Input: part model. Units: mm. Frame: model coordinates. Round coordinates to 2 decimals unless told otherwise and drop trailing zeros. Loops run counter-clockwise (first coordinate to the right, second up) from the corner with the lowest first, then second, coordinate; pieces in that order, holes last. Notation, with made-up numbers: (79, 36.25) -> (97, 36.25) arc R14 ccw to (97, 42.25) -> close; hole circle Ø4 at (50.25, -35.5). An arc over 180 degrees is marked (long way). Answer as a JSON object with one key per item and string values. Group by question number.
Item 1: Section query A-A on z = -255. Return loops of the section in (x, y), and give its area (3 significant figures).
Item 2: Pin query (flat end, axial travel): pin 1 (5.5 mm diameter, centred on y = 12.7, z = 12.7, fed in from +X); pin 2 (4.5 mm diameter, centred on x = 25.4, z = -285.75, fed in from +Y). Return the tip coordinate at first contact, or that it passes through.
Item 3: Material intervals for line 1 (X direction, y = 24.55, z = 31.75); line 2 (Y direction, x = 16, z = -77); line 3 (Y direction, x = 0.85, z = 139.7), sorted ascending. Write a range as [from, to].
Item 4: Section query B-B on y = 19. Return loops of the section in (x, z).
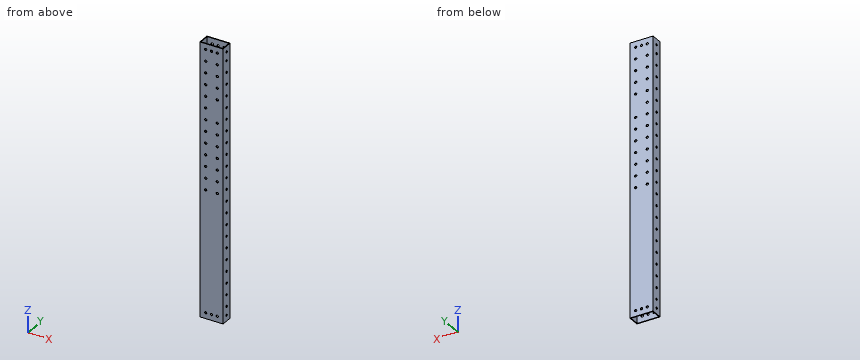
from build123d import *

# Parameters (mm, degrees)
SKETCH1_W           = 50.8
SKETCH1_H           = 25.4
BOSS_EXTRUDE1_DEPTH = 298.45
SHELL1_T            = -1.5875
SKETCH2_R           = 2.4892
CUT_EXTRUDE1_DEPTH  = 304.806192333
SKETCH3_R           = 2.4892
CUT_EXTRUDE2_DEPTH  = 304.806192333
SKETCH4_R           = 2.4892
CUT_EXTRUDE3_DEPTH  = 304.806192333
LPATTERN1_COUNT     = 22
LPATTERN1_PITCH     = 25.4
SKETCH5_R           = 2.4892
CUT_EXTRUDE4_DEPTH  = 304.806192333


with BuildPart() as part:
    # Sketch1 → Boss-Extrude1 (new, symmetric)
    with BuildSketch(Plane.XY):
        with Locations((25.4, 12.7)):
            Rectangle(SKETCH1_W, SKETCH1_H)
    extrude(amount=BOSS_EXTRUDE1_DEPTH, both=True)

    # Shell1
    shell1_openings = [part.faces().sort_by_distance(p)[0] for p in [
        (25.4, 12.7, 298.45),
        (25.4, 12.7, -298.45),
    ]]
    offset(amount=SHELL1_T, openings=shell1_openings, kind=Kind.INTERSECTION)

    # Sketch2 → Cut-Extrude1 (cut, through all)
    with BuildSketch(Plane(origin=(0, 25.4, 0), x_dir=(1, 0, 0), z_dir=(0, 1, 0))):
        with Locations(Location((38.1, -285.75, 0), (0, 0, 270))):
            Circle(SKETCH2_R)
        with Locations(Location((25.4, -285.75, 0), (0, 0, 270))):
            Circle(SKETCH2_R)
        with Locations(Location((12.7, -285.75, 0), (0, 0, 270))):
            Circle(SKETCH2_R)
    cut_extrude1 = extrude(amount=-CUT_EXTRUDE1_DEPTH, mode=Mode.SUBTRACT)

    # Sketch3 → Cut-Extrude2 (cut, through all)
    with BuildSketch(Plane(origin=(50.8, 0, 0), x_dir=(0, 0, -1), z_dir=(1, 0, 0))):
        with Locations((-285.75, 12.7)):
            Circle(SKETCH3_R)
    cut_extrude2 = extrude(amount=-CUT_EXTRUDE2_DEPTH, mode=Mode.SUBTRACT)

    # Mirror1: Cut-Extrude1, Cut-Extrude2 across plane
    add(cut_extrude1.mirror(Plane.XY), mode=Mode.SUBTRACT)
    add(cut_extrude2.mirror(Plane.XY), mode=Mode.SUBTRACT)

    # Sketch4 → Cut-Extrude3 (cut, symmetric)
    with BuildSketch(Plane(origin=(50.8, 0, 0), x_dir=(0, 0, -1), z_dir=(1, 0, 0))):
        with Locations(Location((-266.7, 12.7, 0), (0, 0, 180))):
            Circle(SKETCH4_R)
    cut_extrude3 = extrude(amount=CUT_EXTRUDE3_DEPTH, both=True, mode=Mode.SUBTRACT)

    # LPattern1: Cut-Extrude3 ×22
    with Locations(*[(0, 0, -i * LPATTERN1_PITCH) for i in range(1, LPATTERN1_COUNT)]):
        add(cut_extrude3, mode=Mode.SUBTRACT)

    # Sketch5 → Cut-Extrude4 (cut, through all)
    with BuildSketch(Plane.XZ):
        with Locations(Location((12.7, 158.75, 0), (0, 0, 270))):
            Circle(SKETCH5_R)
        with Locations(Location((12.7, 184.15, 0), (0, 0, 270))):
            Circle(SKETCH5_R)
        with Locations(Location((38.1, 184.15, 0), (0, 0, 270))):
            Circle(SKETCH5_R)
        with Locations(Location((38.1, 209.55, 0), (0, 0, 270))):
            Circle(SKETCH5_R)
        with Locations(Location((12.7, 209.55, 0), (0, 0, 270))):
            Circle(SKETCH5_R)
        with Locations(Location((12.7, 234.95, 0), (0, 0, 270))):
            Circle(SKETCH5_R)
        with Locations(Location((38.1, 234.95, 0), (0, 0, 270))):
            Circle(SKETCH5_R)
        with Locations(Location((38.1, 260.35, 0), (0, 0, 270))):
            Circle(SKETCH5_R)
        with Locations(Location((12.7, 260.35, 0), (0, 0, 270))):
            Circle(SKETCH5_R)
        with Locations(Location((12.7, 31.75, 0), (0, 0, 270))):
            Circle(SKETCH5_R)
        with Locations(Location((38.1, 31.75, 0), (0, 0, 270))):
            Circle(SKETCH5_R)
        with Locations(Location((12.7, 57.15, 0), (0, 0, 270))):
            Circle(SKETCH5_R)
        with Locations(Location((38.1, 57.15, 0), (0, 0, 270))):
            Circle(SKETCH5_R)
        with Locations(Location((12.7, 82.55, 0), (0, 0, 270))):
            Circle(SKETCH5_R)
        with Locations(Location((38.1, 82.55, 0), (0, 0, 270))):
            Circle(SKETCH5_R)
        with Locations(Location((38.1, 107.95, 0), (0, 0, 270))):
            Circle(SKETCH5_R)
        with Locations(Location((38.1, 133.35, 0), (0, 0, 270))):
            Circle(SKETCH5_R)
        with Locations(Location((12.7, 107.95, 0), (0, 0, 270))):
            Circle(SKETCH5_R)
        with Locations(Location((12.7, 133.35, 0), (0, 0, 270))):
            Circle(SKETCH5_R)
        with Locations(Location((38.1, 6.35, 0), (0, 0, 270))):
            Circle(SKETCH5_R)
        with Locations(Location((38.1, -19.05, 0), (0, 0, 270))):
            Circle(SKETCH5_R)
        with Locations(Location((12.7, -19.05, 0), (0, 0, 270))):
            Circle(SKETCH5_R)
        with Locations(Location((12.7, 6.35, 0), (0, 0, 270))):
            Circle(SKETCH5_R)
    extrude(amount=-CUT_EXTRUDE4_DEPTH, mode=Mode.SUBTRACT)


solid = part.part
Solved:
{
 "1": {"outline": "(0, 0) -> (50.8, 0) -> (50.8, 25.4) -> (0, 25.4) -> close; hole (1.59, 1.59) -> (49.21, 1.59) -> (49.21, 23.81) -> (1.59, 23.81) -> close", "area": "232 mm²"},
 "2": {"pin 1": "x = 50.8", "pin 2": "through"},
 "3": {"line 1": "[0, 10.21], [15.19, 35.61], [40.59, 50.8]", "line 2": "[0, 1.59], [23.81, 25.4]", "line 3": "[0, 10.21], [15.19, 25.4]"},
 "4": {"outline": "(0, -298.45) -> (1.59, -298.45) -> (1.59, 298.45) -> (0, 298.45) -> close; (49.21, -298.45) -> (50.8, -298.45) -> (50.8, 298.45) -> (49.21, 298.45) -> close"}
}
